from build123d import *

# Parameters (mm, degrees)
SKETCH_1_W          = 140
SKETCH_1_H          = 300
EXTRUDE_1_DEPTH     = 4
SKETCH_2_W          = 6
SKETCH_2_H          = 300
EXTRUDE_2_DEPTH     = 80
FILLET_1_R          = 140
SKETCH_3_W          = 65
SKETCH_3_H          = 65
EXTRUDE_3_DEPTH     = 1
SKETCH_4_R          = 3.5
SKETCH_4_R_2        = 10
CUT_EXTRUDE_1_DEPTH = 185.122242002
EXTRUDE_START       = 76
EXTRUDE_1_2_DEPTH   = 76
SKETCH_16_R         = 3.5
CUT_EXTRUDE_6_DEPTH = 20


with BuildPart() as part:
    # Эскиз1 → Extrude 1 (new body)
    with BuildSketch(Plane(origin=(0, 0, 0), x_dir=(1, 0, 0), z_dir=(0, 1, 0))):
        Rectangle(SKETCH_1_W, SKETCH_1_H)
    extrude(amount=EXTRUDE_1_DEPTH)

    # Эскиз2 → Бобышка-Вытянуть2 (add)
    with BuildSketch(Plane(origin=(0, 0, 0), x_dir=(1, 0, 0), z_dir=(0, 1, 0))):
        with Locations((73, 0)):
            Rectangle(SKETCH_2_W, SKETCH_2_H)
    extrude(amount=EXTRUDE_2_DEPTH)

    # Скругление1
    fillet_1_edges = [part.edges().sort_by_distance(p)[0] for p in [
        (-70, 2, -150),
        (-70, 2, 150),
    ]]
    fillet(fillet_1_edges, radius=FILLET_1_R)

    # Эскиз3 → Бобышка-Вытянуть3 (add)
    with BuildSketch(Plane(origin=(0, 4, 0), x_dir=(1, 0, 0), z_dir=(0, 1, 0))):
        Rectangle(SKETCH_3_W, SKETCH_3_H)
    extrude(amount=EXTRUDE_3_DEPTH)

    # Эскиз4 → Вырез-Вытянуть1 (cut, through all)
    with BuildSketch(Plane(origin=(0, 5, 0), x_dir=(1, 0, 0), z_dir=(0, 1, 0))):
        with Locations(Location((-25, 25, 0), (0, 0, 270))):
            Circle(SKETCH_4_R)
        with Locations(Location((25, 25, 0), (0, 0, 270))):
            Circle(SKETCH_4_R)
        with Locations(Location((-25, -25, 0), (0, 0, 270))):
            Circle(SKETCH_4_R)
        with Locations(Location((25, -25, 0), (0, 0, 270))):
            Circle(SKETCH_4_R)
        with Locations(Location((0, 0, 0), (0, 0, 270))):
            Circle(SKETCH_4_R_2)
    extrude(amount=-CUT_EXTRUDE_1_DEPTH, mode=Mode.SUBTRACT)

    # Эскиз9 → Extrude 1 2 (add)
    with BuildSketch(Plane(origin=(0, 4, 0), x_dir=(1, 0, 0), z_dir=(0, 1, 0)).offset(EXTRUDE_START)):
        with BuildLine():
            ThreePointArc((70, 147), (-26.873629023, 106.873629023), (-67, 10))
            Line((-67, 10), (-67, -10))
            ThreePointArc((-67, -10), (-26.873629023, -106.873629023), (70, -147))
            Line((70, -147), (70, -150))
            ThreePointArc((70, -150), (-28.994949366, -108.994949366), (-70, -10))
            Line((-70, -10), (-70, 10))
            ThreePointArc((-70, 10), (-28.994949366, 108.994949366), (70, 150))
            Line((70, 150), (70, 147))
        make_face()
    extrude(amount=-EXTRUDE_1_2_DEPTH)

    # Эскиз16 → Вырез-Вытянуть6 (cut)
    with BuildSketch(Plane(origin=(76, 0, 0), x_dir=(0, 0, -1), z_dir=(1, 0, 0))):
        with Locations((0, 65)):
            Circle(SKETCH_16_R)
        with Locations((0, 15)):
            Circle(SKETCH_16_R)
        with Locations((125, 65)):
            Circle(SKETCH_16_R)
        with Locations((-125, 65)):
            Circle(SKETCH_16_R)
        with Locations((-125, 15)):
            Circle(SKETCH_16_R)
        with Locations((125, 15)):
            Circle(SKETCH_16_R)
    extrude(amount=-CUT_EXTRUDE_6_DEPTH, mode=Mode.SUBTRACT)


solid = part.part
Model file for the job. Use its own axes, mm. A direction names the side the tool comes from. Give positions to 0.01 mm unless a question says otherwise; leave off trailing zeros. Order: outer loops, then holes, each group sorted by start corner. A loop starts at its lowest first (then second) coordinate and runs counter-clockwise, first axis right, second up. Notation, with made-up numbers: (-14.5, -1) - (8.5, -1) arc R9 cw to (8.5, 6) - close; hole circle Ø4 at (-4.75, 22). An arc over 180 degrees is marked (long way). One line per item, written item: value.
Item 1: Slice it at D-D (x = 25). List the corners of the cut face in (y, z).
Response values:
outline: (0, -142.57) - (80, -142.57) - (80, -139.4) - (4, -139.4) - (4, -32.5) - (5, -32.5) - (5, -28.5) - (0, -28.5) - close; (0, -21.5) - (5, -21.5) - (5, 21.5) - (0, 21.5) - close; (0, 28.5) - (5, 28.5) - (5, 32.5) - (4, 32.5) - (4, 139.4) - (80, 139.4) - (80, 142.57) - (0, 142.57) - close
Item 2: Wall check: line 1 (Y direction, x = 71.9, z = 0); line 2 (X direction, y = 47, z = 7); line 3 (Y direction, x = 28, z = 50.5). Give the ranges that are in metal, low to high.
Response values:
line 1: 0 to 11.5, 18.5 to 61.5, 68.5 to 80
line 2: -70 to -67, 70 to 76
line 3: 0 to 4
Item 3: Slice it at C-C (y = 29). List the corners of the cut face in (x, z).
Response values:
outline: (-70, -10) arc R140 ccw to (70, -150) - (76, -150) - (76, 150) - (70, 150) arc R140 ccw to (-70, 10) - close; hole (-67, -10) arc R137 ccw to (70, -147) - (70, 147) arc R137 ccw to (-67, 10) - close
Item 4: Pin check, flat tips, straight feed: pin 1 Ø1 at (y, z) = (22.5, 100.5) entering from -X; pin 2 Ø2 at (x, y) = (-1.5, 48) entering from +Z; pin 3 Ø4 at (x, y) = (45.5, 63.5) entering from +Z. Stop position of each tip, or through.
Response values:
pin 1: x = -37.24
pin 2: z = 130.95
pin 3: z = 148.18
Item 5: Slice it at A-A (z = 0). List the corners of the cut face in (x, y).
Response values:
outline: (-70, 0) - (-10, 0) - (-10, 5) - (-32.5, 5) - (-32.5, 4) - (-67, 4) - (-67, 80) - (-70, 80) - close; (10, 0) - (76, 0) - (76, 11.5) - (70, 11.5) - (70, 4) - (32.5, 4) - (32.5, 5) - (10, 5) - close; (70, 18.5) - (76, 18.5) - (76, 61.5) - (70, 61.5) - close; (70, 68.5) - (76, 68.5) - (76, 80) - (70, 80) - close
Item 6: Slice it at B-B (y = 15). List the corners of the cut face in (x, z), then the cut area to 3 significant figures.
Response values:
outline: (-70, -10) arc R140 ccw to (70, -150) - (76, -150) - (76, -128.5) - (70, -128.5) - (70, -147) arc R137 cw to (-67, -10) - (-67, 10) arc R137 cw to (70, 147) - (70, 128.5) - (76, 128.5) - (76, 150) - (70, 150) arc R140 ccw to (-70, 10) - close; (70, -121.5) - (76, -121.5) - (76, -3.5) - (70, -3.5) - close; (70, 3.5) - (76, 3.5) - (76, 121.5) - (70, 121.5) - close
area: 3,040 mm2
Item 7: Tool access for faces 1 (the flat face through (70, 41, 2)), 2 (the cylindrical face through (-22.05, 2.54, -23.12)), 3 (the cylindrical face through (73.042, 11.583, 0.759)): list every direction of +Z, -Z, +X, -X, +Y, -Y with a clear straight run to the whole face (end or side of a thin tool).
Response values:
face 1: +Y
face 2: +Y, -Y
face 3: +X
Item 8: Two-plate mould, pull along Z, no slides. Class faces 4 (the flat face through (73, 39, 150)), 5 (the cylindrical face through (73.04, 66.05, 121.66)), 6 (the flat face through (-70, 41, 0)): released by +Z, released by -Z, zero draft, split by the parting line, or undercut.
Response values:
face 4: released by +Z
face 5: undercut
face 6: zero draft
